For this review, take the finished solid that the model builds, in its own axes (mm). A direction names the side the tool comes from. Give positions to 0.01 mm unless a question says otherwise; leave off trailing zeros. Write each loop counter-clockwise with the first axis right and the second up, starting at its lowest first coordinate (ties: lowest second). Pieces come first, ordered by that corner, then holes.
1) We need section A-A on x = 591. Give the boundary of the cut face in (y, z), and give its area (3 significant figures).
2) Wall thickness on line 1 along Z through (x, y) = (72, 12.5); line 2 along Z through (x, y) = (291.5, 14.5): over which ranges is each line inside the solid? List them lowest first.
3) For P1, Ø2.5, axis at x = 450, z = 7.5, coming from the +Y side, flat-tipped, find the tip position at first contact; note if it passes through.
4) Draft analysis for pull direction Y (two halves, no side actions). For faces 1 (the face through (311, 15, 7)), 2 (the face through (311, 0, 7)), 3 (the face through (319, 7, 1.2)), state which applies: pulls with the +Y half, pulls with the -Y half, needs draft (parallel to the pull), parting line crosses it, or undercut.
5) Machinability: for faces 4 (the face through (319, 1.2, 8)), 5 (the face through (311, 8, 0)), which of the approach directions +Z, -Z, +X, -X, +Y, -Y give a long, thin tool a straight path to every point of the face, cutting with its end or side? Answer none if there is none.
from build123d import *

# Parameters (mm, degrees)
SKETCH_1_W          = 630
SKETCH_1_H          = 15
SKETCH_1_R          = 1.5
EXTRUDE_1_DEPTH     = 15
SKETCH_3_R          = 1.5
CUT_EXTRUDE_1_DEPTH = 631.357041684
SKETCH_4_W          = 12.6
SKETCH_4_H          = 12.6
CUT_EXTRUDE_2_DEPTH = 631.357041684
SKETCH_5_R          = 1.5
CUT_EXTRUDE_3_DEPTH = 631.357041684


with BuildPart() as part:
    # ｽｹｯﾁ1 → ﾎﾞｽ - 押し出し1 (new body)
    with BuildSketch(Plane.XY):
        with Locations((315, 7.5)):
            Rectangle(SKETCH_1_W, SKETCH_1_H)
        with Locations((7.5, 7.5)):
            Circle(SKETCH_1_R, mode=Mode.SUBTRACT)
        with Locations((622.5, 7.5)):
            Circle(SKETCH_1_R, mode=Mode.SUBTRACT)
        with Locations((152.5, 7.5)):
            Circle(SKETCH_1_R, mode=Mode.SUBTRACT)
        with Locations((477.5, 7.5)):
            Circle(SKETCH_1_R, mode=Mode.SUBTRACT)
    extrude(amount=EXTRUDE_1_DEPTH)

    # ｽｹｯﾁ3 → ｶｯﾄ - 押し出し1 (cut, through all)
    with BuildSketch(Plane(origin=(0, 15, 0), x_dir=(1, 0, 0), z_dir=(0, 1, 0))):
        with Locations(Location((30, -7.5, 0), (0, 0, 270))):
            Circle(SKETCH_3_R)
        with Locations(Location((600, -7.5, 0), (0, 0, 270))):
            Circle(SKETCH_3_R)
        with Locations(Location((180, -7.5, 0), (0, 0, 270))):
            Circle(SKETCH_3_R)
        with Locations(Location((450, -7.5, 0), (0, 0, 270))):
            Circle(SKETCH_3_R)
    extrude(amount=-CUT_EXTRUDE_1_DEPTH, mode=Mode.SUBTRACT)

    # ｽｹｯﾁ4 → ｶｯﾄ - 押し出し2 (cut, through all)
    with BuildSketch(Plane(origin=(630, 0, 0), x_dir=(0, 0, -1), z_dir=(1, 0, 0))):
        with Locations((-7.5, 7.5)):
            Rectangle(SKETCH_4_W, SKETCH_4_H)
    extrude(amount=-CUT_EXTRUDE_2_DEPTH, mode=Mode.SUBTRACT)

    # ｽｹｯﾁ5 → ｶｯﾄ - 押し出し3 (cut, through all)
    with BuildSketch(Plane(origin=(0, 15, 0), x_dir=(1, 0, 0), z_dir=(0, 1, 0))):
        with Locations(Location((291.5, -7.5, 0), (0, 0, 270))):
            Circle(SKETCH_5_R)
        with Locations(Location((338.5, -7.5, 0), (0, 0, 270))):
            Circle(SKETCH_5_R)
    extrude(amount=-CUT_EXTRUDE_3_DEPTH, mode=Mode.SUBTRACT)


solid = part.part
Results list:
1. outline: (0, 0) - (15, 0) - (15, 15) - (0, 15) - close; hole (1.2, 1.2) - (13.8, 1.2) - (13.8, 13.8) - (1.2, 13.8) - close
1. area: 66.2 mm2
2. line 1: z = 0 to 1.2, 13.8 to 15
2. line 2: z = 0 to 6, 9 to 15
3. P1: passes through
4. face 1: pulls with the +Y half
4. face 2: pulls with the -Y half
4. face 3: undercut
5. face 4: +X, -X
5. face 5: -Z, +X, -X, +Y, -Y
